Could you check a few things on this model? Use its own coordinates, in mm. Give positions to 0.01 mm unless a question says otherwise; leave off trailing zeros. Loops run counter-clockwise (first coordinate to the right, second up) from the corner with the lowest first, then second, coordinate; pieces in that order, holes last. Notation, with made-up numbers: M -34,-15 L -5,-15 A13 cw -5,2 Z; hole C 14,72.5 d2. An arc over 180 degrees is marked long. Return JSON: item names as keys, results as strings. Group by question number.
1. If we mould it in two halves opening along X, with no side actions, what happens to faces 1 (the flat face through (0, -27, 16)), 2 (the cylindrical face through (25.31, -27.3, 30.83)), 3 (the cylindrical face through (22.935, -31.312, 16.557))? For each: +X half, -X half, draft (parallel to the pull), parting line (faces both ways), or undercut.
2. For pin 1 (1 mm diameter, centred on x = 6.5, z = 18, fed in from -Y), with a flat end and sliding along its axis, tell me the tip position at first contact or that it passes through.
3. Please list where these lines run through material, in increasing order: line 1 (X direction, y = -23, z = 10); line 2 (Z direction, x = 12.25, y = -30.5); line 3 (X direction, y = -24, z = 11).
4. If we section it at C-C (x = 23.5): Write out the boundary of the cut face in (y, z).
5. If we section it at B-B (x = 2.75): Write out the boundary of the cut face in (y, z), plus the area to 3 significant figures.
6. If we section it at A-A (y = -19): Write out the boundary of the cut face in (x, z) (3 decimals), plus the area to 3 significant figures.
```python
from build123d import *

# Parameters (mm, degrees)
F0_W     = 26.8379747868
F0_H     = 32.2756916285
F1_DEPTH = 53.848
F2_R     = 10.4478277996
F3_DEPTH = 43.688
F7_D     = 19.05
F7_DEPTH = 44.45
F7_TIP   = 5.7231973962
F8_R     = 5.08


# Not quite as in the source:
# - the program builds the solid bodies; features that only make, move or delete a surface that nothing else refers to are left out


with BuildPart() as f1:
    # F0 (on Front) → F1 (new body)
    with BuildSketch(Plane.XZ):
        with Locations((13.4189873934, 16.1378458142)):
            Rectangle(F0_W, F0_H)
    extrude(amount=F1_DEPTH)

    # F2 (on face) → F3 (join)
    with BuildSketch(Plane.XZ.offset(53.848)):
        with Locations((11.908470653, 14.5087121055)):
            Circle(F2_R)
    extrude(amount=-F3_DEPTH)

    # F7
    with Locations(Plane.XZ.offset(53.848)):
        with Locations((13.4189873934, 16.1378458142)):
            Hole(F7_D / 2, depth=F7_DEPTH)
            with Locations((0, 0, -(F7_DEPTH + F7_TIP / 2))):  # 118° drill point
                Cone(0, F7_D / 2, F7_TIP, mode=Mode.SUBTRACT)

    # F8
    f8_edges = [f1.edges().sort_by_distance(p)[0] for p in [
        (0, -26.924, 32.275692),
        (26.837975, -26.924, 32.275692),
        (26.837975, -26.924, 0),
        (0, -26.924, 0),
    ]]
    fillet(f8_edges, radius=F8_R)


solid = f1.part
```
Answer:
{
 "1": {"face 1": "-X half", "face 2": "+X half", "face 3": "undercut"},
 "2": {"pin 1": "stops at y = -8.28"},
 "3": {"line 1": "x = 0 to 6.14, 20.7 to 26.84", "line 2": "z = 0 to 6.68, 25.59 to 32.28", "line 3": "x = 0 to 5.4, 21.44 to 26.84"},
 "4": {"outline": "M -53.85,0.31 L 0,0.31 L 0,31.97 L -53.85,31.97 Z"},
 "5": {"outline": "M -53.85,0.57 L 0,0.57 L 0,31.71 L -53.85,31.71 Z", "area": "1,680 mm²"},
 "6": {"outline": "M 0,5.08 A5.08 ccw 5.08,0 L 21.758,0 A5.08 ccw 26.838,5.08 L 26.838,27.196 A5.08 ccw 21.758,32.276 L 5.08,32.276 A5.08 ccw 0,27.196 Z; hole C 13.419,16.138 d19.05", "area": "559 mm²"}
}
